from build123d import *

# Parameters (mm, degrees)
SKETCH1_R           = 3.75
BOSS_EXTRUDE1_DEPTH = 6
SKETCH2_R           = 1.5
CUT_EXTRUDE1_DEPTH  = 39
FILLET1_R           = 10


with BuildPart() as part:
    # Sketch1 → Boss-Extrude1 (new body)
    with BuildSketch(Plane.XY):
        with BuildLine():
            Line((0, 12), (10, 12))
            Line((10, 12), (10, 14))
            Line((10, 14), (0, 14))
            ThreePointArc((0, 14), (-9.050345568, 10.681350341), (-13.809987388, 2.2987493))
            ThreePointArc((-13.809987388, 2.2987493), (-22.82117325, -4.444834248), (-11.937810072, -7.313596289))
            ThreePointArc((-11.937810072, -7.313596289), (-6.841405263, -12.214547639), (0, -14))
            Line((0, -14), (10, -14))
            Line((10, -14), (10, -12))
            Line((10, -12), (0, -12))
            ThreePointArc((0, -12), (-12, 0), (0, 12))
        make_face()
        with Locations((-16.686449258, -3.249986332)):
            Circle(SKETCH1_R, mode=Mode.SUBTRACT)
    extrude(amount=BOSS_EXTRUDE1_DEPTH)

    # Sketch2 → Cut-Extrude1 (cut)
    with BuildSketch(Plane(origin=(0, 14, 0), x_dir=(1, 0, 0), z_dir=(0, 1, 0))):
        with Locations(Location((5, -3, 0), (0, 0, 180))):
            Circle(SKETCH2_R)
    extrude(amount=-CUT_EXTRUDE1_DEPTH, mode=Mode.SUBTRACT)

    # Fillet1
    fillet1_edges = [part.edges().sort_by_distance(p)[0] for p in [
        (-11.937810072, -7.313596289, 3),
        (-13.809987388, 2.2987493, 3),
    ]]
    fillet(fillet1_edges, radius=FILLET1_R)


solid = part.part
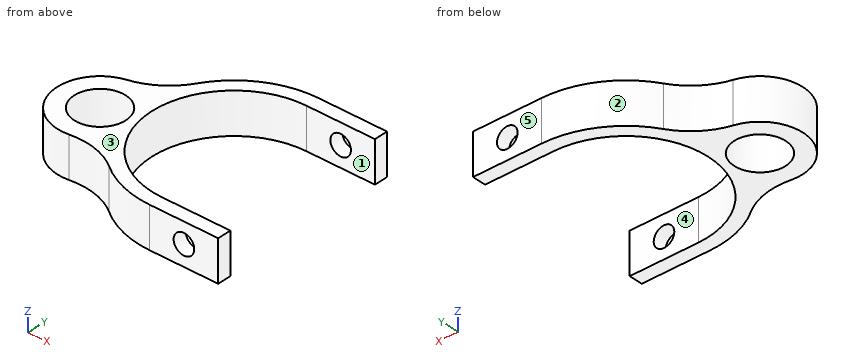
Work out the finished part from the listing and answer in its coordinate system (mm). Face numbers are marked on the shaded views. A direction names the side the tool comes from. Give positions to 0.01 mm unless a question says otherwise; leave off trailing zeros. Write each loop counter-clockwise with the first axis right and the second up, starting at its lowest first coordinate (ties: lowest second). Pieces come first, ordered by that corner, then holes. Notation, with made-up numbers: (52, -22.5) - (106, -22.5) arc R10 ccw to (106, -7.5) - close; hole circle Ø8 at (-20.5, -6). An arc over 180 degrees is marked (long way). One line per item, written item: value. Start each with the question number.
1. Consider probe 1 along Y at (x, z) = (2.5, 2.5); probe 2 along Z at (x, y) = (5, -12.4); probe 3 along Y at (x, z) = (-15, 3). Determine where each line is inside the solid, lowest interval first.
2. Find section C-C (x = -7.5). Write down the section's boundary in (y, z).
3. Find section B-B (y = -1). Write down the section's boundary in (x, z), then the cut area to 3 significant figures.
4. For a pull along Y with two mould halves and no side action, classify the marked faces 1, 2 and 3 as +Y half, -Y half, draft (parallel to the pull), parting line (faces both ways), or undercut.
5. For the marked faces 4 and 5, determine the directions among +Z, -Z, +X, -X, +Y, -Y from which every point of the face is accessible in a straight line to the end or side of a thin tool.
6. Find section A-A (x = 5). Write down the section's boundary in (y, z), then the cut area to 3 significant figures.
7. Given pin 1 (2 mm diameter, centred on y = 4, z = 5, fed in from +X); pin 2 (5 mm diameter, centred on x = -6.5, y = 4.5, fed in from -Z), each flat-ended and moving along its own axis, determine where each tip first touches the part or whether it passes through.
8. Find section D-D (z = 4). State how many separate pieces and enclosed holes the cut face has, then the cut area to 3 significant figures.
Geometry results:
1. probe 1: -14 to -12, 12 to 14
1. probe 2: 0 to 1.5, 4.5 to 6
1. probe 3: -9.34 to -6.6, 0.1 to 4.17
2. outline: (-11.82, 0) - (-9.37, 0) - (-9.37, 6) - (-11.82, 6) - close; (9.37, 0) - (11.82, 0) - (11.82, 6) - (9.37, 6) - close
3. outline: (-22.52, 0) - (-19.69, 0) - (-19.69, 6) - (-22.52, 6) - close; (-13.69, 0) - (-11.96, 0) - (-11.96, 6) - (-13.69, 6) - close
3. area: 27.4 mm2
4. face 1: undercut
4. face 2: +Y half
4. face 3: draft
5. face 4: +Z, -Z, +X
5. face 5: +Z, -Z, +X, -X, +Y
6. outline: (-14, 0) - (-12, 0) - (-12, 1.5) - (-14, 1.5) - close; (-14, 4.5) - (-12, 4.5) - (-12, 6) - (-14, 6) - close; (12, 0) - (14, 0) - (14, 1.5) - (12, 1.5) - close; (12, 4.5) - (14, 4.5) - (14, 6) - (12, 6) - close
6. area: 12.0 mm2
7. pin 1: x = -10.91
7. pin 2: through
8. separate pieces: 3
8. enclosed holes: 1
8. area: 180 mm2
